Work out the finished part from the listing and answer in its coordinate system (mm). A direction names the side the tool comes from. Round coordinates to 2 decimals unless told otherwise and drop trailing zeros. Loops run counter-clockwise (first coordinate to the right, second up) from the corner with the lowest first, then second, coordinate; pieces in that order, holes last.
```python
from build123d import *

# Parameters (mm, degrees)
BOSS_EXTRUDE1_DEPTH = 5.5
SKETCH4_W           = 2
SKETCH4_H           = 1
CUT_EXTRUDE2_DEPTH  = 110
SKETCH5_R           = 10
CUT_EXTRUDE3_DEPTH  = 110
CUT_EXTRUDE4_START  = -4
CUT_EXTRUDE4_DEPTH  = 100
FILLET3_R           = 5.5
FILLET4_R           = 2.75
BOSS_EXTRUDE2_START = -29
SKETCH7_R           = 2
BOSS_EXTRUDE2_DEPTH = 10
BOSS_EXTRUDE3_START = -69
SKETCH7_3_R         = 2
BOSS_EXTRUDE3_DEPTH = 10
CUT_EXTRUDE5_DEPTH  = 155.389928428


with BuildPart() as part:
    # Sketch1 → Boss-Extrude1 (new body)
    with BuildSketch(Plane(origin=(0, 0, 0), x_dir=(1, 0, 0), z_dir=(0, 1, 0))):
        Polygon((0, 110), (4, 110), (4, 100), (104, 100), (104, 110), (108, 110), (108, 0), (0, 0), align=None)
    extrude(amount=BOSS_EXTRUDE1_DEPTH)

    # Sketch4 → Cut-Extrude2 (cut)
    with BuildSketch(Plane(origin=(0, 0, -110), x_dir=(-1, 0, 0), z_dir=(0, 0, -1))):
        with Locations((-3, 0.5)):
            Rectangle(SKETCH4_W, SKETCH4_H)
        with Locations((-3, 5)):
            Rectangle(SKETCH4_W, SKETCH4_H)
        with Locations((-105, 5)):
            Rectangle(SKETCH4_W, SKETCH4_H)
        with Locations((-105, 0.5)):
            Rectangle(SKETCH4_W, SKETCH4_H)
    extrude(amount=-CUT_EXTRUDE2_DEPTH, mode=Mode.SUBTRACT)

    # Sketch5 → Cut-Extrude3 (cut)
    with BuildSketch(Plane(origin=(0, 5.5, 0), x_dir=(1, 0, 0), z_dir=(0, 1, 0))):
        with Locations(Location((54, 50, 0), (0, 0, 270))):
            Circle(SKETCH5_R)
        with BuildLine():
            Line((41.269180349, 41.158267646), (9.5, 9.389087297))
            Line((9.5, 9.389087297), (9.5, 90.610912703))
            Line((9.5, 90.610912703), (41.269180349, 58.841732354))
            ThreePointArc((41.269180349, 58.841732354), (38.5, 50), (41.269180349, 41.158267646))
        make_face()
        with BuildLine():
            Line((98.5, 90.610912703), (98.5, 9.389087297))
            Line((98.5, 9.389087297), (66.730819651, 41.158267646))
            ThreePointArc((66.730819651, 41.158267646), (69.5, 50), (66.730819651, 58.841732354))
            Line((66.730819651, 58.841732354), (98.5, 90.610912703))
        make_face()
        with BuildLine():
            Line((45.158267646, 62.730819651), (16.389087297, 91.5))
            Line((16.389087297, 91.5), (91.610912703, 91.5))
            Line((91.610912703, 91.5), (62.841732354, 62.730819651))
            ThreePointArc((62.841732354, 62.730819651), (54, 65.5), (45.158267646, 62.730819651))
        make_face()
        with BuildLine():
            Line((16.389087297, 8.5), (91.610912703, 8.5))
            Line((91.610912703, 8.5), (62.841732354, 37.269180349))
            ThreePointArc((62.841732354, 37.269180349), (54, 34.5), (45.158267646, 37.269180349))
            Line((45.158267646, 37.269180349), (16.389087297, 8.5))
        make_face()
    extrude(amount=-CUT_EXTRUDE3_DEPTH, mode=Mode.SUBTRACT)

    # Sketch6 → Cut-Extrude4 (cut)
    with BuildSketch(Plane(origin=(108, 0, 0), x_dir=(0, 0, -1), z_dir=(1, 0, 0)).offset(CUT_EXTRUDE4_START)):
        Polygon((0, 0), (5.5, 5.5), (0, 5.5), align=None)
        Polygon((100, 5.5), (100, 0), (94.5, 5.5), align=None)
    extrude(amount=-CUT_EXTRUDE4_DEPTH, mode=Mode.SUBTRACT)

    # Fillet3
    fillet3_edges = [part.edges().sort_by_distance(p)[0] for p in [
        (16.389087297, 2.75, -91.5),
        (91.610912703, 2.75, -91.5),
        (9.5, 2.75, -9.389087297),
        (9.5, 2.75, -90.610912703),
        (98.5, 2.75, -90.610912703),
        (98.5, 2.75, -9.389087297),
        (16.389087297, 2.75, -8.5),
        (91.610912703, 2.75, -8.5),
    ]]
    fillet(fillet3_edges, radius=FILLET3_R)

    # Fillet4
    fillet4_edges = [part.edges().sort_by_distance(p)[0] for p in [
        (62.841732354, 2.75, -62.730819651),
        (45.158267646, 2.75, -62.730819651),
        (41.269180349, 2.75, -58.841732354),
        (41.269180349, 2.75, -41.158267646),
        (66.730819651, 2.75, -41.158267646),
        (66.730819651, 2.75, -58.841732354),
        (45.158267646, 2.75, -37.269180349),
        (62.841732354, 2.75, -37.269180349),
    ]]
    fillet(fillet4_edges, radius=FILLET4_R)

    # Sketch7 → Boss-Extrude2 (add)
    with BuildSketch(Plane(origin=(108, 0, 0), x_dir=(0, 0, -1), z_dir=(1, 0, 0)).offset(BOSS_EXTRUDE2_START)):
        with BuildLine():
            Line((100, 0), (97, 0))
            Line((97, 0), (97, -1.854248689))
            ThreePointArc((97, -1.854248689), (101.645751311, -8.145751311), (100, -0.5))
            Line((100, -0.5), (100, 0))
        make_face()
        with Locations((100, -4.5)):
            Circle(SKETCH7_R, mode=Mode.SUBTRACT)
    extrude(amount=-BOSS_EXTRUDE2_DEPTH)

    # Sketch7_3 → Boss-Extrude3 (add)
    with BuildSketch(Plane(origin=(108, 0, 0), x_dir=(0, 0, -1), z_dir=(1, 0, 0)).offset(BOSS_EXTRUDE3_START)):
        with BuildLine():
            Line((100, 0), (97, 0))
            Line((97, 0), (97, -1.854248689))
            ThreePointArc((97, -1.854248689), (101.645751311, -8.145751311), (100, -0.5))
            Line((100, -0.5), (100, 0))
        make_face()
        with Locations((100, -4.5)):
            Circle(SKETCH7_3_R, mode=Mode.SUBTRACT)
    extrude(amount=-BOSS_EXTRUDE3_DEPTH)

    # Sketch9 → Cut-Extrude5 (cut, through all)
    with BuildSketch(Plane(origin=(108, 0, 0), x_dir=(0, 0, -1), z_dir=(1, 0, 0))):
        with BuildLine():
            Line((110, -2), (115, -2))
            Line((115, -2), (115, 18))
            Line((115, 18), (95, 18))
            Line((95, 18), (95, 13))
            ThreePointArc((95, 13), (105.606601718, 8.606601718), (110, -2))
        make_face()
    extrude(amount=-CUT_EXTRUDE5_DEPTH, mode=Mode.SUBTRACT)


solid = part.part
```
1. Given pin 1 (2 mm diameter, centred on x = 107, z = -56.5, fed in from -Y); pin 2 (5 mm diameter, centred on x = 32.5, y = -4, fed in from -Z); pin 3 (0.6 mm diameter, centred on x = 72.5, y = -0.5, fed in from -Z), each flat-ended and moving along its own axis, determine where each tip first touches the part or whether it passes through.
Answer key:
pin 1: stops at y = 0
pin 2: stops at z = -104
pin 3: stops at z = -101.52
2. Find section B-B (y = -4.5). Write down the section's boundary in (x, z).
Answer key:
outline: (29, -104) - (39, -104) - (39, -102) - (29, -102) - close; (29, -98) - (39, -98) - (39, -96) - (29, -96) - close; (69, -104) - (79, -104) - (79, -102) - (69, -102) - close; (69, -98) - (79, -98) - (79, -96) - (69, -96) - close
3. Which of the six approach directions +Z, -Z, +X, -X, +Y, -Y give full straight-line access (tool end or side, diameter ignored) to faces 4 (the face through (66, 5.5, -51)), 5 (the face through (39, -3, -98)), 6 (the face through (54, 3, -91.5))?
Answer key:
face 4: +Z, -Z, +X, -X, +Y
face 5: +Z, -Z, -Y
face 6: +Y, -Y
4. Find section A-A (x = 54). Write down the section's boundary in (y, z).
Answer key:
outline: (0, -100) - (5.5, -94.5) - (5.5, -91.5) - (0, -91.5) - close; (0, -65.5) - (5.5, -65.5) - (5.5, -60) - (0, -60) - close; (0, -40) - (5.5, -40) - (5.5, -34.5) - (0, -34.5) - close; (0, -8.5) - (5.5, -8.5) - (5.5, -5.5) - (0, 0) - close
5. Determine the mould class of faces 1 (the face through (106, 3, 0)), 2 (the face through (24.62, 2.71, -11.81)), 3 (the face through (108, 3, -56)) for opening direction X: +X half, -X half, draft (parallel to the pull), parting line (faces both ways), or undercut.
Answer key:
face 1: draft
face 2: undercut
face 3: +X half
6. Find section D-D (x = 17.5). Write down the section's boundary in (y, z).
Answer key:
outline: (0, -100) - (5.5, -94.5) - (5.5, -82.23) - (0, -82.23) - close; (0, -17.77) - (5.5, -17.77) - (5.5, -5.5) - (0, 0) - close
7. Find section C-C (z = -50). Give the number of separate pieces and of enclosed holes in the cut face, then the cut area to 3 significant figures.
Answer key:
separate pieces: 4
enclosed holes: 0
area: 157 mm2
8. Consider probe 1 along X at (y, z) = (0.75, -93.5); probe 2 along X at (y, z) = (2, -50); probe 3 along Z at (x, y) = (80.5, 5) (3 decimals). Determine where each line is inside the solid, lowest interval first.
Answer key:
probe 1: x = 0 to 2, 4 to 104, 106 to 108
probe 2: x = 0 to 9.5, 38.5 to 44, 64 to 69.5, 98.5 to 108
probe 3: z = -95 to -91.055, -80.389 to -72.611, -27.389 to -19.611, -8.945 to -5
